```python
from build123d import *

# Parameters (mm, degrees)
BOSS_EXTRUDE1_DEPTH = 3.175
SKETCH4_R           = 2.54
CUT_EXTRUDE3_DEPTH  = 4.175
FILLET1_R           = 5.08


with BuildPart() as part:
    # Sketch1 → Boss-Extrude1 (new body)
    with BuildSketch(Plane.XY):
        Polygon((-38.1, 50.8), (-25.4, 50.8), (-25.4, 12.7), (25.4, 12.7), (25.4, 50.8), (38.1, 50.8), (38.1, -50.8), (25.4, -50.8), (25.4, -12.7), (-25.4, -12.7), (-25.4, -50.8), (-38.1, -50.8), align=None)
    extrude(amount=BOSS_EXTRUDE1_DEPTH)

    # Sketch4 → Cut-Extrude3 (cut, through all)
    with BuildSketch(Plane.XY.offset(3.175)):
        with Locations((-31.75, 44.45)):
            Circle(SKETCH4_R)
        with Locations((-31.75, 6.35)):
            Circle(SKETCH4_R)
        with Locations((31.75, 6.35)):
            Circle(SKETCH4_R)
        with Locations((31.75, 44.45)):
            Circle(SKETCH4_R)
        with Locations((-31.75, -6.35)):
            Circle(SKETCH4_R)
        with Locations((31.75, -6.35)):
            Circle(SKETCH4_R)
        with Locations((31.75, -44.45)):
            Circle(SKETCH4_R)
        with Locations((-31.75, -44.45)):
            Circle(SKETCH4_R)
    extrude(amount=-CUT_EXTRUDE3_DEPTH, mode=Mode.SUBTRACT)

    # Fillet1
    fillet1_edges = [part.edges().sort_by_distance(p)[0] for p in [
        (25.4, -12.7, 1.5875),
        (-25.4, -12.7, 1.5875),
        (-25.4, 12.7, 1.5875),
        (25.4, 12.7, 1.5875),
    ]]
    fillet(fillet1_edges, radius=FILLET1_R)


solid = part.part
```
Design review of the part built by this model. Coordinates are the model's own, in mm. A direction names the side the tool comes from. Coordinates: 2 decimals unless noted, no trailing zeros. Write each loop counter-clockwise with the first axis right and the second up, starting at its lowest first coordinate (ties: lowest second). Pieces come first, ordered by that corner, then holes.
1) To check wall thickness, follow L1, parallel to Y at x = -31.75, z = 1.8; L2, parallel to X at y = 6, z = 1.8; L3, parallel to X at y = 30.5, z = 0.6. State the ranges of each line that lie inside material, in increasing order.
2) Insertion check: pin 1 (1 mm diameter, centred on x = -9.5, z = 2, fed in from -Y); pin 2 (1 mm diameter, centred on x = -4, z = 1.5, fed in from +Y). Each pin has a flat end and moves straight along its axis. Give the tip position at first contact, or say it passes through.
3) Add section B-B (x = -31.75). Write out the cut boundary in (y, z) (3 decimals), plus the area to 3 significant figures.
4) Add section D-D (y = 6.35). Write out the cut boundary in (x, z) (3 decimals).
5) Add section C-C (z = 0.75). State how many separate pieces and enclosed holes the cut face has, plus the area to 3 significant figures.
6) Machinability: for faces 1 (the cylindrical face through (31.2, -46.93, 1.61)), 2 (the flat face through (0, -12.7, 2)), 3 (the cylindrical face through (-23.951, 14.228, 1.61)), which of the approach directions +Z, -Z, +X, -X, +Y, -Y give a long, thin tool a straight path to every point of the face, cutting with its end or side? Answer none if there is none.
7) Add section A-A (y = 36.5). Write out the cut boundary in (x, z) (3 decimals).
8) Mouldability with a two-part tool opening along Y and no side actions: class faces 4 (the flat face through (-32, -50.8, 2)), 5 (the flat face through (32, 50.8, 2)), 6 (the cylindrical face through (-32.08, 46.97, 1.61)) as +Y half, -Y half, draft (parallel to the pull), parting line (faces both ways), or undercut.
Check result:
1. L1: y = -50.8 to -46.99, -41.91 to -8.89, -3.81 to 3.81, 8.89 to 41.91, 46.99 to 50.8
1. L2: x = -38.1 to -34.27, -29.23 to 29.23, 34.27 to 38.1
1. L3: x = -38.1 to -25.4, 25.4 to 38.1
2. pin 1: stops at y = -12.7
2. pin 2: stops at y = 12.7
3. outline: (-50.8, 0) - (-46.99, 0) - (-46.99, 3.175) - (-50.8, 3.175) - close; (-41.91, 0) - (-8.89, 0) - (-8.89, 3.175) - (-41.91, 3.175) - close; (-3.81, 0) - (3.81, 0) - (3.81, 3.175) - (-3.81, 3.175) - close; (8.89, 0) - (41.91, 0) - (41.91, 3.175) - (8.89, 3.175) - close; (46.99, 0) - (50.8, 0) - (50.8, 3.175) - (46.99, 3.175) - close
3. area: 258 mm2
4. outline: (-38.1, 0) - (-34.29, 0) - (-34.29, 3.175) - (-38.1, 3.175) - close; (-29.21, 0) - (29.21, 0) - (29.21, 3.175) - (-29.21, 3.175) - close; (34.29, 0) - (38.1, 0) - (38.1, 3.175) - (34.29, 3.175) - close
5. separate pieces: 1
5. enclosed holes: 8
5. area: 3,730 mm2
6. face 1: +Z, -Z
6. face 2: +Z, -Z, -Y
6. face 3: +Z, -Z, +Y
7. outline: (-38.1, 0) - (-25.4, 0) - (-25.4, 3.175) - (-38.1, 3.175) - close; (25.4, 0) - (38.1, 0) - (38.1, 3.175) - (25.4, 3.175) - close
8. face 4: -Y half
8. face 5: +Y half
8. face 6: undercut
